Part model, mm, in its own coordinate system. A direction names the side the tool comes from. Round coordinates to 2 decimals unless told otherwise and drop trailing zeros. Write each loop counter-clockwise with the first axis right and the second up, starting at its lowest first coordinate (ties: lowest second). Pieces come first, ordered by that corner, then holes. Notation, with made-up numbers: M 7,-11 L 43,-11 A13 ccw 43,-7 Z; hole C 3.25,-37.5 d9. An arc over 180 degrees is marked long. Use one line per item in the form item = value. Start each with the question number.
Item 1: Cut at B-B, the plane z = 3.85. Give the cut face in (x, y) (3 decimals), then the cut area to 3 significant figures.
Item 2: Mould opens along Y. For faces 1 (the face through (20.488, -21.184, 4.014)), 2 (the face through (-24.33, 4.514, 2.465)), 3 (the face through (-24.299, -44.115, 2.465)) say: +Y half, -Y half, draft (parallel to the pull), parting line (faces both ways), or undercut.
Item 3: Cut at C-C, the plane x = 20.55. Give the cut face in (y, z) (3 decimals).
Item 4: Cut at D-D, the plane y = -33. Give the cut face in (x, z), then the cut area to 3 significant figures.
Item 5: Which spindle directions (+Z, -Z, +X, -X, +Y, -Y) get a long thin tool onto all of the face, cutting with end or side? Do faces 4 (the face through (19.649, -16.924, 1.521)), 5 (the face through (-17, -14, 0)), 6 (the face through (-15.6, -24, 2)). Say none if no direction does.
Item 6: Cut at A-A, the plane y = -13. Give the cut face in (x, z).
Item 7: Flat gauge pins, fed straight in: pin 1 Ø3 at (x, z) = (-3.5, 4) entering from -Y (3 decimals); pin 2 Ø0.9 at (x, z) = (14.5, 1.5) entering from -Y (3 decimals). Where does each tip first touch, or does it go through?
Item 8: Probe L1, parallel to Y at x = -20.55, z = 1.6 (3 decimals); L2, parallel to X at y = -34, z = 4.65; L3, parallel to Y at x = -20.55, z = 4.25 (3 decimals). List the from-to ranges inside material, lowest first.
Autodesk Inventor part; units mm, degrees
ref_plane "YZ Plane" through (0, 0, 0) normal (1, 0, 0) x (0, 1, 0)
ref_plane "XZ Plane" through (0, 0, 0) normal (0, 1, 0) x (-1, 0, 0)
ref_plane "XY Plane" through (0, 0, 0) normal (0, 0, 1) x (1, 0, 0)
sketch "Sketch1" plane through (0, 0, 0) normal (0, 0, 1) x (1, 0, 0)
  circle A0 centre (-21, 1.215) radius 1.4
  circle A1 centre (21, 1.215) radius 1.4
  arc A2 (24.9, 3.115) -> (22.9, 5.115) centre (22.9, 3.115) ccw
  line L0 (22.9, 5.115) -> (-22.9, 5.115)
  arc A3 (-22.9, 5.115) -> (-24.9, 3.115) centre (-22.9, 3.115) ccw
  line L1 (-24.9, 3.115) -> (-24.9, -5.115)
  line L2 (22.8395, -5.115) -> (24.9, -5.115)
  line L3 (24.9, -5.115) -> (24.9, 3.115)
  arc A4 (22.9, -44.685) -> (24.9, -42.685) centre (22.9, -42.685) ccw
  line L4 (24.9, -42.685) -> (24.9, -36.885)
  line L5 (24.9, -36.885) -> (17.1, -36.885)
  line L6 (17.1, -36.885) -> (17.1, -44.685)
  line L7 (17.1, -44.685) -> (22.9, -44.685)
  circle A5 centre (21, -40.785) radius 1.4
  arc A6 (-24.9, -42.685) -> (-22.9, -44.685) centre (-22.9, -42.685) ccw
  line L8 (-22.9, -44.685) -> (-17.1, -44.685)
  line L9 (-17.1, -44.685) -> (-17.1, -36.885)
  line L10 (-17.1, -36.885) -> (-24.9, -36.885)
  line L11 (-24.9, -36.885) -> (-24.9, -42.685)
  circle A7 centre (-21, -40.785) radius 1.4
  line L12 (24.9, 5.115) -> (-24.9, 5.115)
  line L13 (-24.9, 5.115) -> (-24.9, -44.685)
  line L14 (-24.9, -44.685) -> (24.9, -44.685)
  line L15 (24.9, -44.685) -> (24.9, 5.115)
  line L16 (17.1, -2.685) -> (-17.1, -2.685)
  line L17 (-17.1, -2.685) -> (-17.1, -36.885)
  line L18 (-17.1, -36.885) -> (17.1, -36.885)
  line L19 (17.1, -36.885) -> (17.1, -2.685)
  line L20 (17.1, -36.885) -> (17.1, -44.685)
  line L21 (-17.1, -36.885) -> (-17.1, -44.685)
  circle A8 centre (0, 1.415) radius 1.4
  arc A9 (-18.2605, -5.115) -> (-22.8395, -5.115) centre (-20.55, -5.335) ccw
  arc A10 (22.8395, -5.115) -> (18.2605, -5.115) centre (20.55, -5.335) ccw
  circle A11 centre (14.45, 0.765) radius 2.3
  circle A12 centre (-14.45, 0.765) radius 2.3
  line L22 (-24.9, -5.115) -> (-22.8395, -5.115)
  line L23 (-18.2605, -5.115) -> (18.2605, -5.115)
  circle A13 centre (20, -39.785) radius 1.4
  circle A14 centre (-20, -39.785) radius 1.4
  circle A15 centre (-14.45, -40.335) radius 2.3
  circle A16 centre (20.55, -34.235) radius 2.3
  circle A17 centre (-20.55, -34.235) radius 2.3
  circle A18 centre (14.45, -40.335) radius 2.3
  arc A19 (22.9, -44.685) -> (24.9, -42.685) centre (22.9, -42.685) ccw
  line L24 (24.9, -42.685) -> (24.9, -4.885)
  line L25 (24.9, -4.885) -> (22.8055, -4.885)
  line L26 (17.1, -4.885) -> (17.1, -36.885)
  line L27 (17.1, -36.885) -> (-17.1, -36.885)
  line L28 (-17.1, -36.885) -> (-17.1, -4.885)
  line L29 (-22.8055, -4.885) -> (-24.9, -4.885)
  line L30 (-24.9, -4.885) -> (-24.9, -42.685)
  arc A20 (-24.9, -42.685) -> (-22.9, -44.685) centre (-22.9, -42.685) ccw
  line L31 (-22.9, -44.685) -> (22.9, -44.685)
  arc A21 (-22.8055, -4.885) -> (-18.2945, -4.885) centre (-20.55, -5.335) ccw
  arc A22 (18.2945, -4.885) -> (22.8055, -4.885) centre (20.55, -5.335) ccw
  line L32 (18.2945, -4.885) -> (17.1, -4.885)
  line L33 (-17.1, -4.885) -> (-18.2945, -4.885)
  line L34 (17.1, -44.685) -> (15.6, -44.685)
  line L35 (15.6, -44.685) -> (15.6, -2.685)
  line L36 (15.6, -2.685) -> (17.1, -2.685)
  line L37 (17.1, -2.685) -> (17.1, -44.685)
  line L38 (-17.1, -44.685) -> (-15.6, -44.685)
  line L39 (-15.6, -44.685) -> (-15.6, -2.685)
  line L40 (-15.6, -2.685) -> (-17.1, -2.685)
  line L41 (-17.1, -2.685) -> (-17.1, -44.685)
  line L42 (-15, -27.435) -> (15, -27.435)
  line L43 (15, -27.435) -> (15, 0.565)
  line L44 (15, 0.565) -> (-15, 0.565)
  line L45 (-15, 0.565) -> (-15, -27.435)
  circle A23 centre (0, -19.785) radius 6.5
  circle A24 centre (-10, -2.435) radius 2.75
  circle A25 centre (10, -2.435) radius 2.75
  line L46 (15.2, 0.765) -> (15.2, -27.635)
  line L47 (15.2, -27.635) -> (-15.2, -27.635)
  line L48 (-15.2, -27.635) -> (-15.2, 0.765)
  line L49 (-15.2, 0.765) -> (15.2, 0.765)
  point P0 (0, 0)
  point P1 (-20.55, -5.335)
  point P2 (20.55, -5.335)
  point P3 (-20.55, -5.335)
  point P4 (20.55, -5.335)
  point P5 (15.2, -2.685)
  point P6 (-15.2, -2.685)
  point P7 (-12.15, 0.765)
  point P8 (-12.1587, 0.565)
  point P9 (12.1587, 0.565)
  point P10 (12.15, 0.765)
  point P11 (-15.6, -36.885)
  point P12 (15.6, -36.885)
  dimension "d0" = 7.8
  dimension "d23" = 1.5
  dimension "d24" = 1.5
  dimension "d57" = 0.2
extrude "Extrusion1" add sketch "Sketch1" along normal blind 5 contours A0 | A1 | L3 L25 A10 L32 L19 L16 L46 A11 L49 A8 A12 L48 L17 L33 A9 L29 L1 A3 L0 A2 | L3 L2 A10 L25 | L15 L5 L19 L23 A22 L2 | A10 A22 | L4 A4 L7 L6 L5 | A10 L23 L19 L32 | L29 A9 L22 L1 | L6 L14 L35 A18 L18 | L18 L35 L23 L19 | L19 L23 L35 L16 | L22 A21 L23 L17 L10 L13 | A9 A21 | L10 L9 L8 A6 L11 | L33 L17 L23 A9 | L39 A15 L14 L9 L18 | L18 L17 L23 L39 | A18 L35 | L17 L16 L39 L23 | L39 A15 | L46 L49 A11 | A12 L49 L48 | L44 A8 L49 A11 | L49 A8 L44 A12 | L44 A8 L49 | L49 A8 | A5 A13 | A13 A5 | A5 A13 | A7 A14 | A7 A14 | A14 A7 | A16 | A17 picked at (16.0467, -40.1174) picked at (-15.7428, -39.7773)
ref_plane "Arbeitsebene1" through (15.3065, -4.4785, 13.1) normal (0, 0, 1) x (0, 1, 0)
sketch "Skizze3" plane through (15.3065, -4.4785, 13.1) normal (0, 0, 1) x (0, 1, 0)
  line L0 (-0.0065, 32.6065) -> (-30.6065, 32.6065)
  arc A0 (1.9935, 30.6065) -> (-0.0065, 32.6065) centre (-0.0065, 30.6065) ccw
  line L1 (1.9935, 30.6065) -> (1.9935, 0.0065)
  arc A1 (-0.0065, -1.9935) -> (1.9935, 0.0065) centre (-0.0065, 0.0065) ccw
  line L2 (-0.0065, -1.9935) -> (-30.6065, -1.9935)
  arc A2 (-32.6065, 0.0065) -> (-30.6065, -1.9935) centre (-30.6065, 0.0065) ccw
  line L3 (-32.6065, 0.0065) -> (-32.6065, 30.6065)
  arc A3 (-30.6065, 32.6065) -> (-32.6065, 30.6065) centre (-30.6065, 30.6065) ccw
  circle A4 centre (-35.2065, 35.2065) radius 2.4
  circle A5 centre (-35.8565, 29.7565) radius 2.45
  circle A6 centre (-29.7565, 35.8565) radius 2.45
  circle A7 centre (-35.2065, -4.5935) radius 2.4
  circle A8 centre (-35.8565, 0.8565) radius 2.45
  circle A9 centre (-29.7565, -5.2435) radius 2.45
  circle A10 centre (4.5935, 35.2065) radius 2.4
  circle A11 centre (5.2435, 29.7565) radius 2.45
  circle A12 centre (-0.8565, 35.8565) radius 2.45
  circle A13 centre (-0.8565, -5.2435) radius 2.45
  circle A14 centre (5.2435, 0.8565) radius 2.45
  circle A15 centre (4.5935, -4.5935) radius 2.4
  line L4 (-10.3065, -9.6935) -> (7.6935, -9.6935)
  arc A16 (7.6935, -9.6935) -> (9.6935, -7.6935) centre (7.6935, -7.6935) ccw
  line L5 (9.6935, 10.3065) -> (9.6935, -7.6935)
  line L6 (9.6935, 10.3065) -> (10.5197, 10.3065)
  arc A17 (10.9935, 9.9665) -> (10.5197, 10.3065) centre (10.5197, 9.8065) ccw
  arc A18 (10.9935, 9.9665) -> (12.953, 8.3665) centre (12.953, 10.3665) ccw
  line L7 (12.953, 8.3665) -> (13.0935, 8.3665)
  arc A19 (13.0935, 8.3665) -> (15.0935, 10.3665) centre (13.0935, 10.3665) ccw
  line L8 (15.0935, 10.3665) -> (15.0935, 20.2465)
  arc A20 (15.0935, 20.2465) -> (13.0935, 22.2465) centre (13.0935, 20.2465) ccw
  line L9 (13.0935, 22.2465) -> (12.953, 22.2465)
  arc A21 (12.953, 22.2465) -> (10.9935, 20.6465) centre (12.953, 20.2465) ccw
  arc A22 (10.5197, 20.3065) -> (10.9935, 20.6465) centre (10.5197, 20.8065) ccw
  line L10 (10.5197, 20.3065) -> (9.6935, 20.3065)
  line L11 (9.6935, 38.3065) -> (9.6935, 20.3065)
  arc A23 (9.6935, 38.3065) -> (7.6935, 40.3065) centre (7.6935, 38.3065) ccw
  line L12 (7.6935, 40.3065) -> (-10.156, 40.3065)
  line L13 (-10.156, 40.3065) -> (-10.1563, 39.5805)
  arc A24 (-10.1563, 39.5805) -> (-9.9265, 39.2516) centre (-9.8062, 39.5805) ccw
  arc A25 (-8.2165, 37.1473) -> (-9.9265, 39.2516) centre (-10.3665, 37.1472) ccw
  line L14 (-8.2165, 37.1473) -> (-8.2165, 37.007)
  arc A26 (-10.3664, 34.8569) -> (-8.2165, 37.007) centre (-10.3665, 37.0069) ccw
  line L15 (-10.3664, 34.8569) -> (-20.25, 34.8563)
  arc A27 (-22.4012, 37.0074) -> (-20.25, 34.8563) centre (-20.2501, 37.0074) ccw
  line L16 (-22.4012, 37.0074) -> (-22.4012, 37.1472)
  arc A28 (-20.6871, 39.2564) -> (-22.4012, 37.1472) centre (-20.2465, 37.1472) ccw
  arc A29 (-20.6871, 39.2564) -> (-20.4574, 39.5808) centre (-20.8064, 39.5844) ccw
  line L17 (-20.4574, 39.5808) -> (-20.4576, 40.3065)
  line L18 (-20.4576, 40.3065) -> (-38.3065, 40.3065)
  arc A30 (-38.3065, 40.3065) -> (-40.3065, 38.3065) centre (-38.3065, 38.3065) ccw
  line L19 (-40.3065, 20.4571) -> (-40.3065, 38.3065)
  line L20 (-40.3065, 20.4571) -> (-39.5805, 20.4567)
  arc A31 (-39.5805, 20.4567) -> (-39.2516, 20.6865) centre (-39.5805, 20.8069) ccw
  arc A32 (-37.1473, 22.3966) -> (-39.2516, 20.6865) centre (-37.1472, 20.2466) ccw
  line L21 (-37.1473, 22.3966) -> (-37.007, 22.3966)
  arc A33 (-34.8569, 20.2467) -> (-37.007, 22.3966) centre (-37.0069, 20.2466) ccw
  line L22 (-34.8569, 20.2467) -> (-34.8563, 10.3631)
  arc A34 (-37.0074, 8.2119) -> (-34.8563, 10.3631) centre (-37.0074, 10.363) ccw
  line L23 (-37.0074, 8.2119) -> (-37.1472, 8.2119)
  arc A35 (-39.2564, 9.9259) -> (-37.1472, 8.2119) centre (-37.1472, 10.3665) ccw
  arc A36 (-39.2564, 9.9259) -> (-39.5808, 10.1556) centre (-39.5844, 9.8067) ccw
  line L24 (-39.5808, 10.1556) -> (-40.3065, 10.1554)
  line L25 (-40.3065, -7.6935) -> (-40.3065, 10.1554)
  arc A37 (-40.3065, -7.6935) -> (-38.3065, -9.6935) centre (-38.3065, -7.6935) ccw
  line L26 (-38.3065, -9.6935) -> (-20.3065, -9.6935)
  line L27 (-20.3065, -9.6935) -> (-20.3065, -10.5197)
  arc A38 (-20.6465, -10.9935) -> (-20.3065, -10.5197) centre (-20.8065, -10.5197) ccw
  arc A39 (-20.6465, -10.9935) -> (-22.2465, -12.953) centre (-20.2465, -12.953) ccw
  line L28 (-22.2465, -12.953) -> (-22.2465, -13.0935)
  arc A40 (-22.2465, -13.0935) -> (-20.2465, -15.0935) centre (-20.2465, -13.0935) ccw
  line L29 (-20.2465, -15.0935) -> (-10.3665, -15.0935)
  arc A41 (-10.3665, -15.0935) -> (-8.3665, -13.0935) centre (-10.3665, -13.0935) ccw
  line L30 (-8.3665, -13.0935) -> (-8.3665, -12.953)
  arc A42 (-8.3665, -12.953) -> (-9.9665, -10.9935) centre (-10.3665, -12.953) ccw
  arc A43 (-10.3065, -10.5197) -> (-9.9665, -10.9935) centre (-9.8065, -10.5197) ccw
  line L31 (-10.3065, -10.5197) -> (-10.3065, -9.6935)
  circle A44 centre (-15.4065, -5.9935) radius 2.15
  circle A45 centre (5.9935, 15.2065) radius 2.15
  point P0 (4.4785, 15.3065)
hole "Bohrung1" at (-20.55, -34.235, 13.1) at (-20.55, -5.335, 13.1) at (20.55, -5.335, 13.1) at (20.55, -34.235, 13.1) direction (0, 0, -1) diameter 4.6 end through all
sketch "Skizze10" plane through (0, 0, 0) normal (0, 0, -1) x (-1, 0, 0)
  circle A0 centre (-20.55, -19.785) radius 1.4
  circle A1 centre (20.55, -19.785) radius 1.4
  point P0 (0, 0)
hole "Bohrung5" at (20.55, -19.785, 0) at (-20.55, -19.785, 0) direction (0, 0, 1) diameter 2.8 end through all counterbore diameter 6 counterbore depth 3
properties part number "30_Linear_Stage_NEMA11_China_lid_universal_extender_v2"
Model answer:
q1.outline = M -24.9,-42.685 A2 ccw -22.9,-44.685 L -15.6,-44.685 L -15.6,-2.685 L -15.2,-2.685 L -15.2,0.765 L -12.15,0.765 A2.3 cw -12.159,0.565 L 12.159,0.565 A2.3 cw 12.15,0.765 L 15.2,0.765 L 15.2,-2.685 L 15.6,-2.685 L 15.6,-44.685 L 22.9,-44.685 A2 ccw 24.9,-42.685 L 24.9,3.115 A2 ccw 22.9,5.115 L -22.9,5.115 A2 ccw -24.9,3.115 Z; hole C -20.55,-34.235 d4.6; hole C -20.55,-5.335 d4.6; hole C -20.55,-19.785 d2.8; hole C 20.55,-34.235 d4.6; hole C 20.55,-5.335 d4.6; hole C 20.55,-19.785 d2.8
q1.area = 987 mm²
q2.face_1 = undercut
q2.face_2 = +Y half
q2.face_3 = -Y half
q3.outline = M -44.685,0 L -36.535,0 L -36.535,5 L -44.685,5 Z; M -31.935,0 L -22.785,0 L -22.785,3 L -21.185,3 L -21.185,5 L -31.935,5 Z; M -18.385,3 L -16.785,3 L -16.785,0 L -7.635,0 L -7.635,5 L -18.385,5 Z; M -3.035,0 L 5.115,0 L 5.115,5 L -3.035,5 Z
q4.outline = M -24.9,0 L -22.49,0 L -22.49,5 L -24.9,5 Z; M -18.61,0 L -15.6,0 L -15.6,5 L -18.61,5 Z; M 15.6,0 L 18.61,0 L 18.61,5 L 15.6,5 Z; M 22.49,0 L 24.9,0 L 24.9,5 L 22.49,5 Z
q4.area = 54.2 mm²
q5.face_4 = -Z
q5.face_5 = -Z, +X, -X, +Y, -Y
q5.face_6 = +Z, -Z, -Y
q6.outline = M -24.9,0 L -15.6,0 L -15.6,5 L -24.9,5 Z; M 15.6,0 L 24.9,0 L 24.9,5 L 15.6,5 Z
q7.pin_1 = 0.565
q7.pin_2 = 0.765
q8.L1 = -44.685 to -36.535, -31.935 to -22.785, -16.785 to -7.635, -3.035 to 5.115
q8.L2 = -24.9 to -22.84, -18.26 to -15.6, 15.6 to 18.26, 22.84 to 24.9
q8.L3 = -44.685 to -36.535, -31.935 to -21.185, -18.385 to -7.635, -3.035 to 5.115
